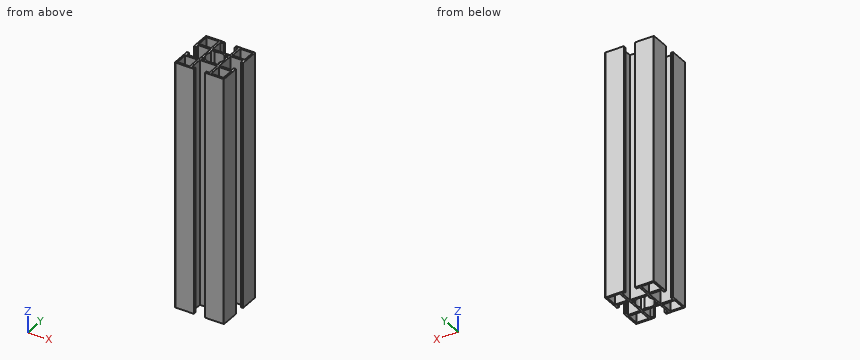
```python
from build123d import *

# Parameters (mm, degrees)
SKETCH1_W                 = 10
SKETCH1_H                 = 10
F_40_X_40A_X_R0_5_1_DEPTH = 200


with BuildPart() as part:
    # Sketch1 → 铝型材 40 X 40A X R0.5(1) (new body)
    with BuildSketch(Plane.YX):
        with BuildLine():
            Line((-19.5, 20), (-4.5, 20))
            Line((-4.5, 20), (-4.5, 18.2))
            Line((-4.5, 18.2), (-7.1, 18.2))
            Line((-7.1, 18.2), (-7.1, 8.2))
            Line((-7.1, 8.2), (7.1, 8.2))
            Line((7.1, 8.2), (7.1, 18.2))
            Line((7.1, 18.2), (4.5, 18.2))
            Line((4.5, 18.2), (4.5, 20))
            Line((4.5, 20), (19.5, 20))
            ThreePointArc((19.5, 20), (19.853553391, 19.853553391), (20, 19.5))
            Line((20, 19.5), (20, 4.5))
            Line((20, 4.5), (18.2, 4.5))
            Line((18.2, 4.5), (18.2, 7.1))
            Line((18.2, 7.1), (8.2, 7.1))
            Line((8.2, 7.1), (8.2, -7.1))
            Line((8.2, -7.1), (18.2, -7.1))
            Line((18.2, -7.1), (18.2, -4.5))
            Line((18.2, -4.5), (20, -4.5))
            Line((20, -4.5), (20, -19.5))
            ThreePointArc((20, -19.5), (19.853553391, -19.853553391), (19.5, -20))
            Line((19.5, -20), (4.5, -20))
            Line((4.5, -20), (4.5, -18.2))
            Line((4.5, -18.2), (7.1, -18.2))
            Line((7.1, -18.2), (7.1, -8.2))
            Line((7.1, -8.2), (-7.1, -8.2))
            Line((-7.1, -8.2), (-7.1, -18.2))
            Line((-7.1, -18.2), (-4.5, -18.2))
            Line((-4.5, -18.2), (-4.5, -20))
            Line((-4.5, -20), (-19.5, -20))
            ThreePointArc((-19.5, -20), (-19.853553391, -19.853553391), (-20, -19.5))
            Line((-20, -19.5), (-20, -4.5))
            Line((-20, -4.5), (-18.2, -4.5))
            Line((-18.2, -4.5), (-18.2, -7.1))
            Line((-18.2, -7.1), (-8.2, -7.1))
            Line((-8.2, -7.1), (-8.2, 7.1))
            Line((-8.2, 7.1), (-18.2, 7.1))
            Line((-18.2, 7.1), (-18.2, 4.5))
            Line((-18.2, 4.5), (-20, 4.5))
            Line((-20, 4.5), (-20, 19.5))
            ThreePointArc((-20, 19.5), (-19.853553391, 19.853553391), (-19.5, 20))
        make_face()
        with BuildLine():
            Line((-4.87903679, 6.434671709), (-4.110433762, 5.66606868))
            ThreePointArc((-4.110433762, 5.66606868), (0, 7), (4.110433762, 5.66606868))
            Line((4.110433762, 5.66606868), (4.87903679, 6.434671709))
            ThreePointArc((4.87903679, 6.434671709), (6.434671709, 6.434671709), (6.434671709, 4.87903679))
            Line((6.434671709, 4.87903679), (5.66606868, 4.110433762))
            ThreePointArc((5.66606868, 4.110433762), (7, 0), (5.66606868, -4.110433762))
            Line((5.66606868, -4.110433762), (6.434671709, -4.87903679))
            ThreePointArc((6.434671709, -4.87903679), (6.434671709, -6.434671709), (4.87903679, -6.434671709))
            Line((4.87903679, -6.434671709), (4.110433762, -5.66606868))
            ThreePointArc((4.110433762, -5.66606868), (0, -7), (-4.110433762, -5.66606868))
            Line((-4.110433762, -5.66606868), (-4.87903679, -6.434671709))
            ThreePointArc((-4.87903679, -6.434671709), (-6.434671709, -6.434671709), (-6.434671709, -4.87903679))
            Line((-6.434671709, -4.87903679), (-5.66606868, -4.110433762))
            ThreePointArc((-5.66606868, -4.110433762), (-7, 0), (-5.66606868, 4.110433762))
            Line((-5.66606868, 4.110433762), (-6.434671709, 4.87903679))
            ThreePointArc((-6.434671709, 4.87903679), (-6.434671709, 6.434671709), (-4.87903679, 6.434671709))
        make_face(mode=Mode.SUBTRACT)
        with Locations((-13.7, 13.7)):
            Rectangle(SKETCH1_W, SKETCH1_H, mode=Mode.SUBTRACT)
        with Locations((13.7, 13.7)):
            Rectangle(SKETCH1_W, SKETCH1_H, mode=Mode.SUBTRACT)
        with Locations((13.7, -13.7)):
            Rectangle(SKETCH1_W, SKETCH1_H, mode=Mode.SUBTRACT)
        with Locations((-13.7, -13.7)):
            Rectangle(SKETCH1_W, SKETCH1_H, mode=Mode.SUBTRACT)
    extrude(amount=F_40_X_40A_X_R0_5_1_DEPTH)


solid = part.part
```
Build history of the part. All positions in model axes, mm. Coordinates: 2 decimals unless noted, no trailing zeros. Order: outer loops, then holes, each group sorted by start corner. A loop starts at its lowest first (then second) coordinate and runs counter-clockwise, first axis right, second up. Notation, with made-up numbers: M 87.25,85.5 L 112.25,85.5 A20 cw 112.25,91.5 Z; hole C -38.5,3 d9. An arc over 180 degrees is marked long. One line per question, with ' | ' between items. Start each with the question number.
1. Cut at C-C (y = -2). Write the cut outline in (x, z), plus the area to 3 significant figures.
2. Cut at D-D (z = -52). Count the separate pieces of the cut face and the enclosed holes in it, plus the area to 3 significant figures.
3. Wall check: line 1 along X through (y, z) = (-15, -187); line 2 along Y through (x, z) = (-8.5, -12.5). Give the ranges that are in metal, low to high. Write a range as [from, to].
4. Cut at A-A (x = 11.5). Write the cut outline in (y, z).
The answers:
1) outline: M -8.2,-200 L -6.71,-200 L -6.71,0 L -8.2,0 Z; M 6.71,-200 L 8.2,-200 L 8.2,0 L 6.71,0 Z | area: 597 mm2
2) separate pieces: 1 | enclosed holes: 5 | area: 396 mm2
3) line 1: x = [-20, -18.7], [-8.7, -7.1], [7.1, 8.7], [18.7, 20] | line 2: y = [-20, -7.1], [7.1, 20]
4) outline: M -20,-200 L -18.7,-200 L -18.7,0 L -20,0 Z; M -8.7,-200 L -7.1,-200 L -7.1,0 L -8.7,0 Z; M 7.1,-200 L 8.7,-200 L 8.7,0 L 7.1,0 Z; M 18.7,-200 L 20,-200 L 20,0 L 18.7,0 Z
